Geometry check sheet. Reference: the model listing, model coordinates, mm. Face numbers are marked on the shaded views. A direction names the side the tool comes from. Coordinates: 2 decimals unless noted, no trailing zeros. Loops run counter-clockwise (first coordinate to the right, second up) from the corner with the lowest first, then second, coordinate; pieces in that order, holes last.
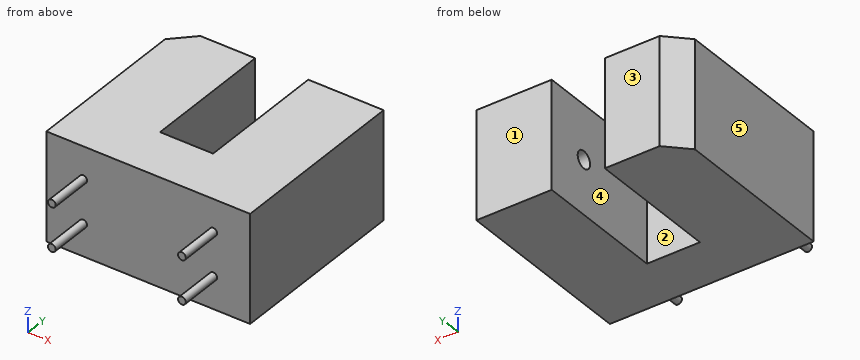
from build123d import *

# Parameters (mm, degrees)
SKETCH1_W           = 11.9
SKETCH1_H           = 6.3
BOSS_EXTRUDE1_DEPTH = 3.1
SKETCH2_W           = 4.4
SKETCH2_H           = 6.3
BOSS_EXTRUDE2_DEPTH = 7.7
SKETCH3_R           = 0.5
CUT_EXTRUDE1_DEPTH  = 1
CHAMFER1_SIZE       = 1.2
SKETCH4_R           = 0.225
BOSS_EXTRUDE3_DEPTH = 2.54


with BuildPart() as part:
    # Sketch1 → Boss-Extrude1 (new body)
    with BuildSketch(Plane(origin=(0, 0, 0), x_dir=(1, 0, 0), z_dir=(0, 1, 0))):
        Rectangle(SKETCH1_W, SKETCH1_H)
    extrude(amount=BOSS_EXTRUDE1_DEPTH)

    # Sketch2 → Boss-Extrude2 (add)
    with BuildSketch(Plane(origin=(0, 3.1, 0), x_dir=(1, 0, 0), z_dir=(0, 1, 0))):
        with Locations((-3.75, 0)):
            Rectangle(SKETCH2_W, SKETCH2_H)
        with Locations((3.75, 0)):
            Rectangle(SKETCH2_W, SKETCH2_H)
    extrude(amount=BOSS_EXTRUDE2_DEPTH)

    # Sketch3 → Cut-Extrude1 (cut)
    with BuildSketch(Plane.ZY.offset(-1.55)):
        with Locations((0, 8.2)):
            Circle(SKETCH3_R)
    extrude(amount=-CUT_EXTRUDE1_DEPTH, mode=Mode.SUBTRACT)

    # Chamfer1
    chamfer1_edges = [part.edges().sort_by_distance(p)[0] for p in [
        (-5.95, 10.8, 0),
    ]]
    chamfer(chamfer1_edges, length=CHAMFER1_SIZE)

    # Sketch4 → Boss-Extrude3 (add)
    with BuildSketch(Plane.XZ):
        with Locations(Location((-3.8, 1.27, 0), (0, 0, 90))):
            Circle(SKETCH4_R)
        with Locations(Location((-3.8, -1.27, 0), (0, 0, 90))):
            Circle(SKETCH4_R)
        with Locations(Location((3.8, 1.27, 0), (0, 0, 90))):
            Circle(SKETCH4_R)
        with Locations(Location((3.8, -1.27, 0), (0, 0, 90))):
            Circle(SKETCH4_R)
    extrude(amount=BOSS_EXTRUDE3_DEPTH)


solid = part.part
(1) Sectioned sample at B-B on y = 3.5. Record the cut outline in (x, z), and give its area (3 significant figures).
Findings:
outline: (-5.95, -3.15) - (-1.55, -3.15) - (-1.55, 3.15) - (-5.95, 3.15) - close; (1.55, -3.15) - (5.95, -3.15) - (5.95, 3.15) - (1.55, 3.15) - close
area: 55.4 mm2
(2) Gauge pin test, flat end, axial feed: pin 1 Ø1 at (x, z) = (-0.5, 0) entering from +Y. Record the tip position at first contact, or that the pin passes through.
Findings:
pin 1: stops at y = 3.1
(3) Sectioned sample at A-A on z = 0. Record the cut outline in (x, y), and give its area (3 significant figures).
Findings:
outline: (-5.95, 0) - (5.95, 0) - (5.95, 10.8) - (1.55, 10.8) - (1.55, 8.7) - (2.55, 8.7) - (2.55, 7.7) - (1.55, 7.7) - (1.55, 3.1) - (-1.55, 3.1) - (-1.55, 10.8) - (-4.75, 10.8) - (-5.95, 9.6) - close
area: 103 mm2
(4) Draft check along X on the marked faces 3, 4 and 5. Enter one of: +X half, -X half, draft (parallel to the pull), parting line (faces both ways), or undercut.
Findings:
face 3: draft
face 4: undercut
face 5: -X half
(5) Access from +Z, -Z, +X, -X, +Y, -Y to the whole of each face (thin tool, end or side, straight path). Record for the marked faces 1 and 2.
Findings:
face 1: +Z, -Z, +X, -X, +Y
face 2: +Z, -Z, +Y
(6) Sectioned sample at D-D on z = 2.25. Record the cut outline in (x, y).
Findings:
outline: (-5.95, 0) - (5.95, 0) - (5.95, 10.8) - (1.55, 10.8) - (1.55, 3.1) - (-1.55, 3.1) - (-1.55, 10.8) - (-4.75, 10.8) - (-5.95, 9.6) - close
(7) Scan lines: L1, parallel to X at y = 8.5, z = -2.5; L2, parallel to Y at x = 2.35, z = 0. Record each from-to range of solid material in increasing order.
Findings:
L1: x = -5.95 to -1.55, 1.55 to 5.95
L2: y = 0 to 7.7, 8.7 to 10.8
(8) Sectioned sample at C-C on x = 3.8. Record the cut outline in (y, z) (3 decimals).
Findings:
outline: (-2.54, -1.495) - (0, -1.495) - (0, -3.15) - (10.8, -3.15) - (10.8, 3.15) - (0, 3.15) - (0, 1.495) - (-2.54, 1.495) - (-2.54, 1.045) - (0, 1.045) - (0, -1.045) - (-2.54, -1.045) - close
